Here's how the part is built. I have some questions about the finished solid (model axes, mm). Coordinates: 2 decimals unless noted, no trailing zeros. Write each loop counter-clockwise with the first axis right and the second up, starting at its lowest first coordinate (ties: lowest second). Pieces come first, ordered by that corner, then holes.
Item 1: If we section it at D-D (x = 92): Please give me the cut outline in (y, z), then the cut area to 3 significant figures.
Item 2: If we section it at A-A (x = 13.5): Please give me the cut outline in (y, z).
Item 3: If I drill on line 1 (Z direction, x = -50, y = -2.5); line 2 (X direction, y = -3.25, z = 6.5); line 3 (X direction, y = -1.5, z = -4.5), over which ranges is the centre line in solid material (lowest first)?
Item 4: I'm going to push flat-ended pins straight in: pin 1 Ø4 at (x, y) = (34, -1) entering from +Z; pin 2 Ø3 at (y, z) = (-1.5, -1.5) entering from +X; pin 3 Ø6 at (x, y) = (31, 1) entering from +Z; pin 4 Ø1.5 at (x, y) = (39, -0.5) entering from +Z. Where does each tip first touch, or does it pass through?
Item 5: If we section it at C-C (z = 15): Please give me the cut outline in (x, y).
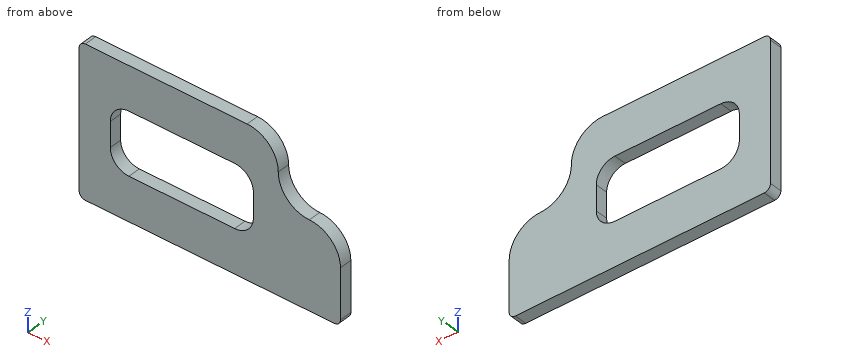
from build123d import *

# Parameters (mm, degrees)
F0_W     = 115
F0_H     = 50
F1_DEPTH = 5
F2_R     = 24.99999
F3_R     = 5
F4_R     = 15


# Not quite as in the source:
# - a fillet or chamfer is up to 0.001 mm smaller than in the source, because OpenCascade refuses the exact size


with BuildPart() as f1:
    # F0 (on Front) → F1 (new body, symmetric)
    with BuildSketch(Plane.XZ):
        Polygon((55, 60), (-105, 60), (-105, -60), (105, -60), (105, 10), (55, 10), align=None)
        with Locations((-22.5, 0)):
            Rectangle(F0_W, F0_H, mode=Mode.SUBTRACT)
    extrude(amount=F1_DEPTH, both=True)

    # F2 (radius 25 in the source; OpenCascade refuses exactly that, so slightly less here)
    f2_edges = [f1.edges().sort_by_distance(p)[0] for p in [
        (55, 0, 10),
        (105, 0, 10),
        (55, 0, 60),
    ]]
    fillet(f2_edges, radius=F2_R)

    # F3
    f3_edges = [f1.edges().sort_by_distance(p)[0] for p in [
        (105, 0, -60),
        (-105, 0, -60),
        (-105, 0, 60),
    ]]
    fillet(f3_edges, radius=F3_R)

    # F4
    f4_edges = [f1.edges().sort_by_distance(p)[0] for p in [
        (-80, 0, -25),
        (35, 0, -25),
        (35, 0, 25),
        (-80, 0, 25),
    ]]
    fillet(f4_edges, radius=F4_R)


solid = f1.part
Answer list:
1. outline: (-5, -60) - (5, -60) - (5, 6.93) - (-5, 6.93) - close
1. area: 669 mm2
2. outline: (-5, -60) - (5, -60) - (5, -25) - (-5, -25) - close; (-5, 25) - (5, 25) - (5, 60) - (-5, 60) - close
3. line 1: z = -60 to -25, 25 to 60
3. line 2: x = -105 to -80, 35 to 92.76
3. line 3: x = -105 to -80, 35 to 102.69
4. pin 1: stops at z = 59.92
4. pin 2: stops at x = 101.93
4. pin 3: stops at z = 60
4. pin 4: stops at z = 58.6
5. outline: (-105, -5) - (-79.14, -5) - (-79.14, 5) - (-105, 5) - close; (34.14, -5) - (65, -5) - (65, 5) - (34.14, 5) - close
